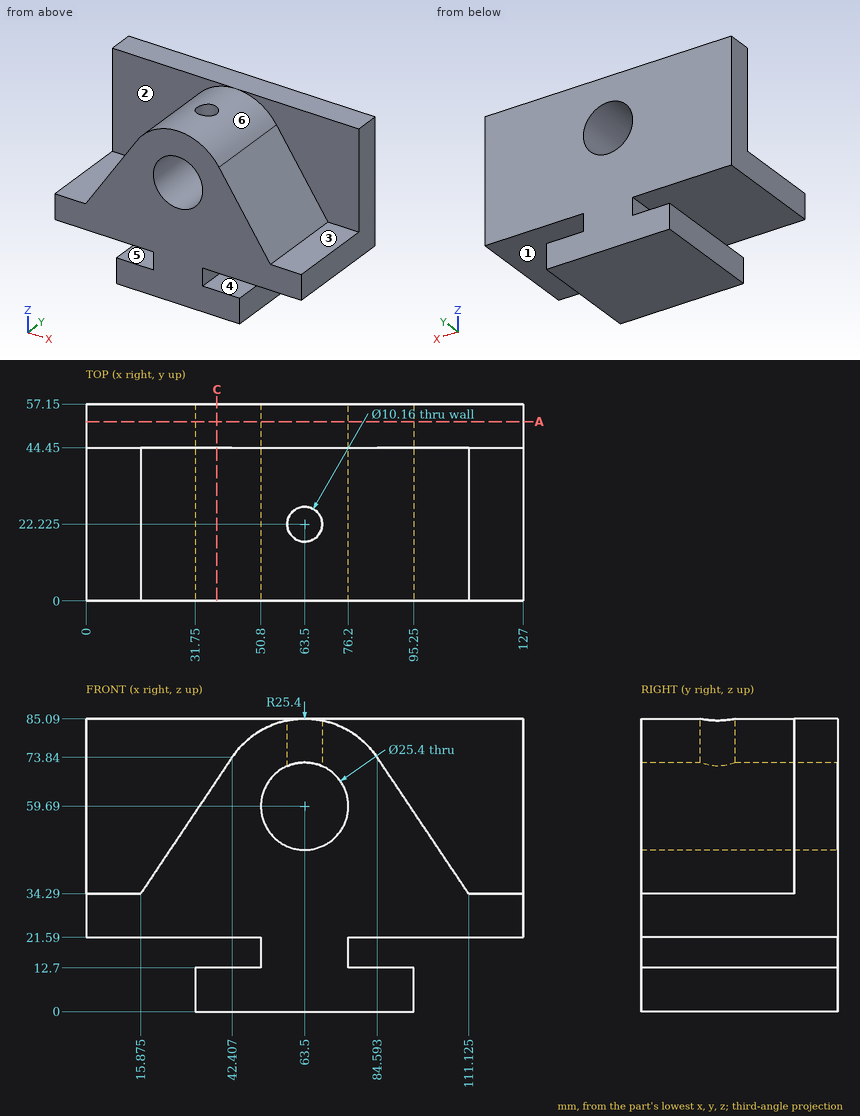
Here's the drawing with two shaded views (mm, measured from the low corner). I have some questions. A direction names the side the tool comes from. Give positions to 0.01 mm unless a question says otherwise; leave off trailing zeros. Loops run counter-clockwise (first coordinate to the right, second up) from the corner with the lowest first, then second, coordinate; pieces in that order, holes last. Notation, with made-up numbers: M 35.5,-0.75 L 75.5,-0.75 A17 ccw 75.5,20.25 Z; hole C 37.5,22.5 d3. An arc over 180 degrees is marked long. One line per item, written item: value.
1) I'm going to push flat-ended pins straight in: pin 1 (10 mm diameter, centred on y = 16.5, z = 8.5, fed in from +X); pin 2 (15 mm diameter, centred on x = 108.5, z = 66.5, fed in from -Y); pin 3 (5 mm diameter, centred on x = 11, y = 13.5, fed in from +Z). Where does each tip first touch, or does it pass through?
Geometry check:
pin 1: stops at x = 95.25
pin 2: stops at y = 44.45
pin 3: stops at z = 34.29
2) On a 3-axis mill with a long thin cutter (end or side, diameter ignored), from which of +Z, -Z, +X, -X, +Y, -Y can I reach the whole of each face in a straight line? I mean the marked faces 4, 5 and 6. Say none if no direction works.
Geometry check:
face 4: +X, +Y, -Y
face 5: -X, +Y, -Y
face 6: +Z, -Y
3) Thinking about a two-plate mould opening in Z: for the marked faces 1, 2 and 3, which applies, +Z half, -Z half, draft (parallel to the pull), parting line (faces both ways), or undercut?
Geometry check:
face 1: undercut
face 2: draft
face 3: +Z half
4) Imagine slicing it at A-A on y = 52. Write out the boundary of the cut face in (x, z), and give its area (3 significant figures).
Geometry check:
outline: M 0,21.59 L 50.8,21.59 L 50.8,12.7 L 31.75,12.7 L 31.75,0 L 95.25,0 L 95.25,12.7 L 76.2,12.7 L 76.2,21.59 L 127,21.59 L 127,85.09 L 0,85.09 Z; hole C 63.5,59.69 d25.4
area: 8,590 mm²
5) Please list where these lines run through material, in increasing order: line 1 (Z direction, x = 63.5, y = 44); line 2 (X direction, y = 28.5, z = 5); line 3 (Y direction, x = 27, z = 76).
Geometry check:
line 1: z = 0 to 46.99, 72.39 to 85.09
line 2: x = 31.75 to 95.25
line 3: y = 44.45 to 57.15
6) Imagine slicing it at C-C on x = 38. Write out the boundary of the cut face in (y, z), and give its area (3 significant figures).
Geometry check:
outline: M 0,0 L 57.15,0 L 57.15,12.7 L 0,12.7 Z; M 0,21.59 L 57.15,21.59 L 57.15,85.09 L 44.45,85.09 L 44.45,67.27 L 0,67.27 Z
area: 3,560 mm²
